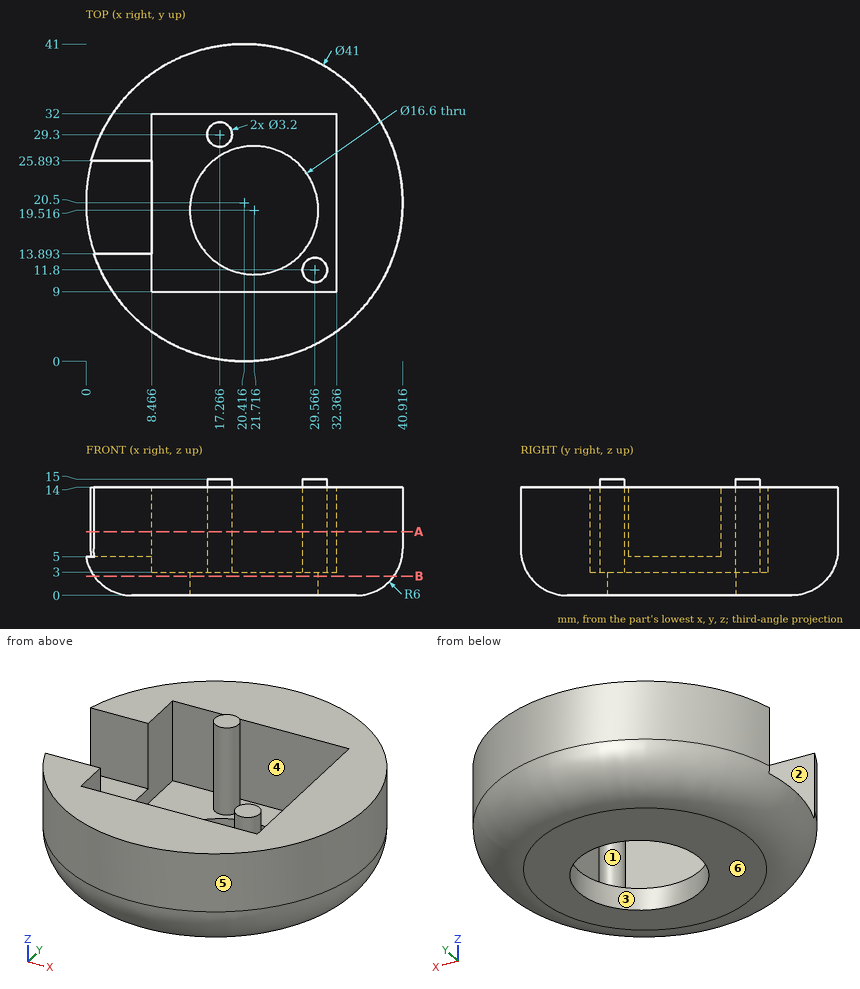
Design review of the part shown in the three views and the two pictorial views. Dimensions are in mm from the part's minimum x, y and z. A direction names the side the tool comes from. Round coordinates to 2 decimals unless told otherwise and drop trailing zeros. Order: outer loops, then holes, each group sorted by start corner. A loop starts at its lowest first (then second) coordinate and runs counter-clockwise, first axis right, second up.
Q1. We need section B-B, the plane z = 2.5. Give the boundary of the cut face in (x, y), plus the area to 3 significant figures.
Findings below:
outline: circle Ø38.75 at (20.42, 20.5); hole circle Ø16.6 at (21.72, 19.52)
area: 963 mm2
Q2. We need section A-A, the plane z = 8.25. Give the boundary of the cut face in (x, y).
Findings below:
outline: (0.64, 25.89) - (8.47, 25.89) - (8.47, 32) - (32.37, 32) - (32.37, 9) - (8.47, 9) - (8.47, 13.89) - (1.01, 13.89) arc R20.5 ccw (long way) to start; circle Ø3.2 at (17.27, 29.3); circle Ø3.2 at (29.57, 11.8)
Q3. Mouldability with a two-part tool opening along Y and no side actions: class the marked faces 4, 5 and 6 as pulls with the +Y half, pulls with the -Y half, needs draft (parallel to the pull), parting line crosses it, or undercut.
Findings below:
face 4: undercut
face 5: parting line crosses it
face 6: needs draft
Q4. Wall thickness on line 1 (Y direction, x = 22.5, z = 12.75); line 2 (X direction, y = 20, z = 9); line 3 (X direction, y = 13.5, z = 9.75) (1 decimal): over which ranges is each line inside the solid? List them lowest first.
Findings below:
line 1: y = 0.11 to 9, 32 to 40.89
line 2: x = 32.37 to 40.91
line 3: x = 1.1 to 8.5, 32.4 to 39.7
Q5. Insertion check: P1, Ø6.5, axis at x = 3, z = 9, coming from the -Y side; P2, Ø3, axis at x = 34, z = 8, coming from the -Y side; P3, Ø3, axis at x = 24.5, z = 9.5, coming from the +Y side. Each pin has a flat end and moves straight along its axis. Give the tip position at first contact, or say it passes through.
Findings below:
P1: stops at y = 5.68
P2: stops at y = 3.94
P3: stops at y = 40.84
Q6. Machinability: for the marked faces 1, 2 and 3, which of the approach directions +Z, -Z, +X, -X, +Y, -Y give a long, thin tool a straight path to every point of the face, cutting with its end or side? Answer none if there is none.
Findings below:
face 1: +Z
face 2: +Z, -X
face 3: +Z, -Z
